Source: CAD feature listing. Evaluate the final solid. Frame: model axes, mm. A direction names the side the tool comes from. Coordinates: 2 decimals unless noted, no trailing zeros. Order: outer loops, then holes, each group sorted by start corner. A loop starts at its lowest first (then second) coordinate and runs counter-clockwise, first axis right, second up. Notation, with made-up numbers: (39, -35) -> (97, -35) arc R32 cw to (97, 4) -> close; hole circle Ø10 at (-9, 87). An arc over 180 degrees is marked (long way). Put each result on its own line as item: value.
from build123d import *

# Parameters (mm, degrees)
BOSS_EXTRUDE1_DEPTH = 100
SKETCH3_W           = 20
SKETCH3_H           = 20
BOSS_EXTRUDE2_DEPTH = 8
SKETCH4_W           = 5
SKETCH4_H           = 100
BOSS_EXTRUDE3_DEPTH = 8
SKETCH5_W           = 5
SKETCH5_H           = 100
BOSS_EXTRUDE4_DEPTH = 8
SKETCH6_R           = 1.75
CUT_EXTRUDE1_DEPTH  = 8
CHAMFER1_SIZE       = 0.5
SKETCH7_W           = 15
SKETCH7_H           = 2
BOSS_EXTRUDE5_DEPTH = 15
SKETCH8_W           = 15
SKETCH8_H           = 2
BOSS_EXTRUDE6_DEPTH = 15
SKETCH9_R           = 2.15
CUT_EXTRUDE2_DEPTH  = 15
CHAMFER2_SIZE       = 1


with BuildPart() as part:
    # Sketch2 → Boss-Extrude1 (new body)
    with BuildSketch(Plane(origin=(0, 0, 0), x_dir=(1, 0, 0), z_dir=(0, 1, 0))):
        Polygon((0, 0), (0, 100), (20, 100), (20, 20), (100, 20), (100, 0), align=None)
    extrude(amount=BOSS_EXTRUDE1_DEPTH)

    # Sketch3 → Boss-Extrude2 (add)
    with BuildSketch(Plane(origin=(0, 100, 0), x_dir=(1, 0, 0), z_dir=(0, 1, 0))):
        with Locations((10, 10)):
            Rectangle(SKETCH3_W, SKETCH3_H)
    extrude(amount=BOSS_EXTRUDE2_DEPTH)

    # Sketch4 → Boss-Extrude3 (add)
    with BuildSketch(Plane(origin=(100, 0, 0), x_dir=(0, 0, -1), z_dir=(1, 0, 0))):
        with Locations((10, 50)):
            Rectangle(SKETCH4_W, SKETCH4_H)
    extrude(amount=BOSS_EXTRUDE3_DEPTH)

    # Sketch5 → Boss-Extrude4 (add)
    with BuildSketch(Plane(origin=(0, 0, -100), x_dir=(-1, 0, 0), z_dir=(0, 0, -1))):
        with Locations((-10, 50)):
            Rectangle(SKETCH5_W, SKETCH5_H)
    extrude(amount=BOSS_EXTRUDE4_DEPTH)

    # Sketch6 → Cut-Extrude1 (cut)
    with BuildSketch(Plane(origin=(0, 100, 0), x_dir=(1, 0, 0), z_dir=(0, 1, 0))):
        with Locations(Location((50, 10, 0), (0, 0, 270))):
            Circle(SKETCH6_R)
        with Locations(Location((10, 50, 0), (0, 0, 270))):
            Circle(SKETCH6_R)
    extrude(amount=-CUT_EXTRUDE1_DEPTH, mode=Mode.SUBTRACT)

    # Chamfer1
    chamfer1_edges = [part.edges().sort_by_distance(p)[0] for p in [
        (50, 100, -11.75),
        (10, 100, -51.75),
    ]]
    chamfer(chamfer1_edges, length=CHAMFER1_SIZE)

    # Sketch7 → Boss-Extrude5 (add)
    with BuildSketch(Plane.XY):
        with Locations((22.5, 1)):
            Rectangle(SKETCH7_W, SKETCH7_H)
        with Locations((77.5, 1)):
            Rectangle(SKETCH7_W, SKETCH7_H)
    extrude(amount=BOSS_EXTRUDE5_DEPTH)

    # Sketch8 → Boss-Extrude6 (add)
    with BuildSketch(Plane.ZY):
        with Locations((-77.5, 1)):
            Rectangle(SKETCH8_W, SKETCH8_H)
        with Locations((-22.5, 1)):
            Rectangle(SKETCH8_W, SKETCH8_H)
    extrude(amount=BOSS_EXTRUDE6_DEPTH)

    # Sketch9 → Cut-Extrude2 (cut)
    with BuildSketch(Plane(origin=(0, 2, 0), x_dir=(1, 0, 0), z_dir=(0, 1, 0))):
        with Locations(Location((-7.5, 77.5, 0), (0, 0, 270))):
            Circle(SKETCH9_R)
        with Locations(Location((-7.5, 22.5, 0), (0, 0, 270))):
            Circle(SKETCH9_R)
        with Locations(Location((22.5, -7.5, 0), (0, 0, 270))):
            Circle(SKETCH9_R)
        with Locations(Location((77.5, -7.5, 0), (0, 0, 270))):
            Circle(SKETCH9_R)
    extrude(amount=-CUT_EXTRUDE2_DEPTH, mode=Mode.SUBTRACT)

    # Chamfer2
    chamfer2_edges = [part.edges().sort_by_distance(p)[0] for p in [
        (-7.5, 0, -79.65),
        (-7.5, 2, -79.65),
        (-7.5, 2, -24.65),
        (22.5, 0, 5.35),
        (22.5, 2, 5.35),
        (77.5, 0, 5.35),
        (77.5, 2, 5.35),
    ]]
    chamfer(chamfer2_edges, length=CHAMFER2_SIZE - 0.0001)  # a hair under: the kernel refuses the full size


solid = part.part
1. Set-up query: faces 4 (the flat face through (10, 104, -20)), 5 (the flat face through (104, 49, -7.5)), 6 (the flat face through (65, 100, -10)). Return all of +Z, -Z, +X, -X, +Y, -Y with unobstructed straight access to the full face (end or side cutting, diameter ignored); none if empty.
Numbers:
face 4: -Z, +X, -X, +Y
face 5: +Z, +X, +Y, -Y
face 6: +Z, -Z, +X, +Y
2. First-contact query: pin 1 (3 mm diameter, centred on y = 76.5, z = -46.5, fed in from -X); pin 2 (12 mm diameter, centred on x = 79, z = 10, fed in from +Y); pin 3 (10 mm diameter, centred on x = 72, z = -6, fed in from +Y). Flat tips, straight axial feed; report the tip coordinate or a pass-through.
Numbers:
pin 1: stops at x = 0
pin 2: stops at y = 2
pin 3: stops at y = 100
3. Pull-direction query (X, two-part tool) for faces 1 (the flat face through (-7, 2, -74)), 2 (the cylindrical face through (48.29, 95.8, -10.38)), 3 (the flat face through (108, 51, -10)); classes: pulls with the +X half, pulls with the -X half, needs draft (parallel to the pull), parting line crosses it, or undercut.
Numbers:
face 1: needs draft
face 2: undercut
face 3: pulls with the +X half
4. Ray query, line 1 along X through (y, z) = (0.45, -22.5); line 2 along Z through (x, y) = (-7, 1); line 3 along X through (y, z) = (97.75, -50). Return the intervals inside material, ascending.
Numbers:
line 1: x = -15 to -9.65, -5.35 to 20
line 2: z = -85 to -79.59, -75.41 to -70, -30 to -24.59, -20.41 to -15
line 3: x = 0 to 8.25, 11.75 to 20
5. Cut plane D-D on z = -10. Output: boundary loops of the cut face in (x, y).
Numbers:
outline: (0, 0) -> (108, 0) -> (108, 100) -> (52.25, 100) -> (51.75, 99.5) -> (51.75, 92) -> (48.25, 92) -> (48.25, 99.5) -> (47.75, 100) -> (20, 100) -> (20, 108) -> (0, 108) -> close
6. Cut plane A-A on z = -22.5. Output: boundary loops of the cut face in (x, y), plus the area to 3 significant figures.
Numbers:
outline: (-15, 0) -> (-9.65, 0) -> (-9.65, 1) -> (-10.65, 2) -> (-15, 2) -> close; (-5.35, 0) -> (20, 0) -> (20, 100) -> (0, 100) -> (0, 2) -> (-4.35, 2) -> (-5.35, 1) -> close
area: 2,020 mm2
7. Cut plane C-C on y = 48. Output: boundary loops of the cut face in (x, z), plus the area to 3 significant figures.
Numbers:
outline: (0, -100) -> (7.5, -100) -> (7.5, -108) -> (12.5, -108) -> (12.5, -100) -> (20, -100) -> (20, -20) -> (100, -20) -> (100, -12.5) -> (108, -12.5) -> (108, -7.5) -> (100, -7.5) -> (100, 0) -> (0, 0) -> close
area: 3,680 mm2
